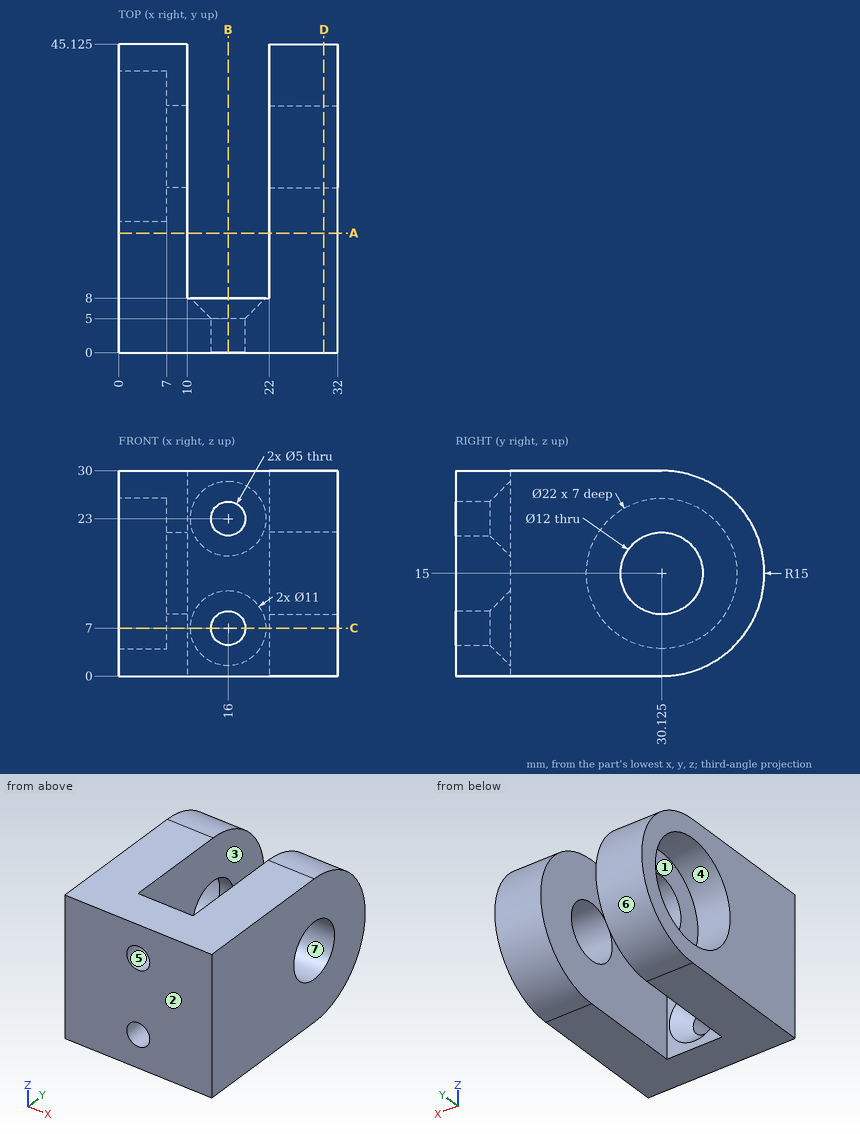
The figure shows three views and two pictorial views of one solid part (mm, origin at its lowest corner). Answer the questions. A direction names the side the tool comes from. Coordinates: 2 decimals unless noted, no trailing zeros. Loops run counter-clockwise (first coordinate to the right, second up) from the corner with the lowest first, then second, coordinate; pieces in that order, holes last.
1) Find section D-D on x = 30. Write down the section's boundary in (y, z) (3 decimals).
2) Determine the mould class of the marked faces 4, 5, 6 and 7 for opening direction Y: pulls with the +Y half, pulls with the -Y half, needs draft (parallel to the pull), parting line crosses it, or undercut.
3) Find section A-A on y = 17.5. Write down the section's boundary in (x, z), then the cut area to 3 significant figures.
4) Find section C-C on z = 7. Write down the section's boundary in (x, y).
5) Flat-ended cylindrical pins translate along their axes: pin 1 Ø11 at (y, z) = (27.5, 17) entering from -X; pin 2 Ø6 at (x, y) = (6.5, 31) entering from -Z; pin 3 Ø4 at (x, z) = (11, 8.5) entering from +Y; pin 4 Ø7 at (y, z) = (30.125, 15) entering from -X. Find the tip coordinate at first contact, or state that the pin passes through.
6) A tool of negligible diameter and unlimited length cuts with its end or side. For the marked faces 1, 2 and 3, from which of +Z, -Z, +X, -X, +Y, -Y can it reach the whole face along a straight path? Write none if from no direction.
7) Find the intervals of material crossed by L1, parallel to Y at x = 27.5, z = 15 (3 decimals); L2, parallel to X at y = 31, z = 24.25; L3, parallel to Y at x = 5, z = 14.5, in increasing order.
8) Find section B-B on x = 16. Write down the section's boundary in (y, z), then the cut area to 3 significant figures.
Values:
1. outline: (0, 0) - (30.125, 0) arc R15 ccw to (30.125, 30) - (0, 30) - close; hole circle Ø12 at (30.125, 15)
2. face 4: undercut
2. face 5: needs draft
2. face 6: pulls with the +Y half
2. face 7: undercut
3. outline: (0, 0) - (10, 0) - (10, 30) - (0, 30) - close; (22, 0) - (32, 0) - (32, 30) - (22, 30) - close
3. area: 600 mm2
4. outline: (0, 0) - (13.5, 0) - (13.5, 5) - (10.5, 8) - (10, 8) - (10, 42.81) - (0, 42.81) - (0, 37.67) - (7, 37.67) - (7, 22.58) - (0, 22.58) - close; (18.5, 0) - (32, 0) - (32, 42.81) - (22, 42.81) - (22, 8) - (21.5, 8) - (18.5, 5) - close
5. pin 1: stops at x = 7
5. pin 2: stops at z = 0
5. pin 3: stops at y = 44.35
5. pin 4: passes through
6. face 1: -X
6. face 2: +Z, -Z, +X, -X, -Y
6. face 3: +Z, -Z, +Y
7. L1: y = 0 to 24.125, 36.125 to 45.125
7. L2: x = 7 to 10, 22 to 32
7. L3: y = 0 to 19.14, 41.11 to 45.12
8. outline: (0, 0) - (8, 0) - (8, 1.5) - (5, 4.5) - (0, 4.5) - close; (0, 9.5) - (5, 9.5) - (8, 12.5) - (8, 17.5) - (5, 20.5) - (0, 20.5) - close; (0, 25.5) - (5, 25.5) - (8, 28.5) - (8, 30) - (0, 30) - close
8. area: 142 mm2
